from build123d import *

# Parameters (mm, degrees)
SKETCH_1_W      = 40
SKETCH_1_H      = 5
SKETCH_1_R      = 1.25
EXTRUDE_1_DEPTH = 4


with BuildPart() as part:
    # 스케치1 → 보스-돌출1 (new body)
    with BuildSketch(Plane(origin=(0, 0, 0), x_dir=(1, 0, 0), z_dir=(0, 1, 0))):
        Rectangle(SKETCH_1_W, SKETCH_1_H)
        Circle(SKETCH_1_R, mode=Mode.SUBTRACT)
        with Locations((15, 0)):
            Circle(SKETCH_1_R, mode=Mode.SUBTRACT)
        with Locations((-15, 0)):
            Circle(SKETCH_1_R, mode=Mode.SUBTRACT)
    extrude(amount=EXTRUDE_1_DEPTH)


solid = part.part
Could you check a few things on this model? Use its own coordinates, in mm. Give positions to 0.01 mm unless a question says otherwise; leave off trailing zeros. Order: outer loops, then holes, each group sorted by start corner. A loop starts at its lowest first (then second) coordinate and runs counter-clockwise, first axis right, second up. Notation, with made-up numbers: (-33.75, 80) -> (7.25, 80) arc R17 ccw to (7.25, 101) -> close; hole circle Ø8 at (12.25, 77). An arc over 180 degrees is marked (long way). Answer in a Markdown table with one row per item. Add a question column.
Item 1: Imagine slicing it at A-A (z = 0). List the corners of the cut face in (x, y) for me, and give its area (3 significant figures).
Item 2: Imagine slicing it at C-C (x = 15). List the corners of the cut face in (y, z) for me, and give its area (3 significant figures).
Item 3: Imagine slicing it at B-B (y = 2.4). List the corners of the cut face in (x, z) for me, and give its area (3 significant figures).
Item 4: Please list where these lines run through material, in increasing order: probe 1 along X at (y, z) = (3.25, 0); probe 2 along Z at (x, y) = (15, 1.05); probe 3 along X at (y, z) = (2.25, 0.5).
Item 5: We'd pull the mould along Z, two halves only. Please class faces 1 (the flat face through (20, 2, 0)), 2 (the cylindrical face through (-16.25, 1.97, -0.05)), 3 (the flat face through (0, 2, -2.5)), 4 (the cylindrical face through (13.75, 1.97, -0.05)): pulls with the +Z half, pulls with the -Z half, needs draft (parallel to the pull), parting line crosses it, or undercut.
Result:
| question | item | result |
|---|---|---|
| 1 | outline | (-20, 0) -> (-16.25, 0) -> (-16.25, 4) -> (-20, 4) -> close; (-13.75, 0) -> (-1.25, 0) -> (-1.25, 4) -> (-13.75, 4) -> close; (1.25, 0) -> (13.75, 0) -> (13.75, 4) -> (1.25, 4) -> close; (16.25, 0) -> (20, 0) -> (20, 4) -> (16.25, 4) -> close |
| 1 | area | 130 mm2 |
| 2 | outline | (0, -2.5) -> (4, -2.5) -> (4, -1.25) -> (0, -1.25) -> close; (0, 1.25) -> (4, 1.25) -> (4, 2.5) -> (0, 2.5) -> close |
| 2 | area | 10.0 mm2 |
| 3 | outline | (-20, -2.5) -> (20, -2.5) -> (20, 2.5) -> (-20, 2.5) -> close; hole circle Ø2.5 at (-15, 0); hole circle Ø2.5 at (0, 0); hole circle Ø2.5 at (15, 0) |
| 3 | area | 185 mm2 |
| 4 | probe 1 | -20 to -16.25, -13.75 to -1.25, 1.25 to 13.75, 16.25 to 20 |
| 4 | probe 2 | -2.5 to -1.25, 1.25 to 2.5 |
| 4 | probe 3 | -20 to -16.15, -13.85 to -1.15, 1.15 to 13.85, 16.15 to 20 |
| 5 | face 1 | needs draft |
| 5 | face 2 | undercut |
| 5 | face 3 | pulls with the -Z half |
| 5 | face 4 | undercut |
